Design review of the part built by this model. Coordinates are the model's own, in mm. A direction names the side the tool comes from. Round coordinates to 2 decimals unless told otherwise and drop trailing zeros. Order: outer loops, then holes, each group sorted by start corner. A loop starts at its lowest first (then second) coordinate and runs counter-clockwise, first axis right, second up. Notation, with made-up numbers: (-8, -30) - (-4, -30) arc R21 ccw to (-4, 2) - close; hole circle Ø9 at (-24, 14.25). An arc over 180 degrees is marked (long way). Write item = value, one per line.
from build123d import *
from build123d import SkipClean  # not in build123d's __all__

# Parameters (mm, degrees)
F0_R     = 26
F1_DEPTH = 8
F2_R     = 26.25
F2_R_2   = 20
F3_DEPTH = 82.5


with BuildPart() as f1:
    # F0 (on Top) → F1 (new body)
    with BuildSketch(Plane.XY):
        Circle(F0_R)
        with BuildLine():
            ThreePointArc((7, 18.7349939952), (19.9390246123, -1.5605439791), (4, -19.5959179423))
            Line((4, -19.5959179423), (2.5, -16.9978417309))
            ThreePointArc((2.5, -16.9978417309), (0, -17.1816769299), (-2.5, -16.9978417309))
            Line((-2.5, -16.9978417309), (-4, -19.5959179423))
            ThreePointArc((-4, -19.5959179423), (-19.9390246123, -1.5605439791), (-7, 18.7349939952))
            Line((-7, 18.7349939952), (-5, 16.4989260177))
            ThreePointArc((-5, 16.4989260177), (0, 17.2452185999), (5, 16.4989260177))
            Line((5, 16.4989260177), (7, 18.7349939952))
        make_face(mode=Mode.SUBTRACT)
    extrude(amount=F1_DEPTH)

    # F2 (on face) → F3 (join)
    with BuildSketch(Plane.XY.offset(8)):
        Circle(F2_R)
        Circle(F2_R_2, mode=Mode.SUBTRACT)
    with SkipClean():  # cleaning this boolean's faces spoils the solid; the shape is the same uncleaned
        extrude(amount=F3_DEPTH)


solid = f1.part
1) Clearance check with flat-ended pins moving along their axes: pin 1 Ø3 at (x, z) = (6, 47.5) entering from -Y; pin 2 Ø4 at (y, z) = (-11, 64.5) entering from +X; pin 3 Ø3 at (y, z) = (3, 35.5) entering from -X. State where each tip first meets the part, or that it passes through.
Findings:
pin_1 = -25.86
pin_2 = 24.66
pin_3 = -26.21
2) For faces 5 (the cylindrical face through (-20.633, -15.821, 3.944)), 6 (the flat face through (-6, -19.3, 90.5)), 7 (the cylindrical face through (0.04, -17.18, 3.94)), 8 (the flat face through (0, -18, 8)), list the 3-axis set-ups (+Z, -Z, +X, -X, +Y, -Y) from which the entire face can be reached by the end or side of a thin tool; tool diameter is ignored.
Findings:
face_5 = -Z
face_6 = +Z, +X, -X, +Y, -Y
face_7 = +Z, -Z
face_8 = +Z
3) We need section A-A on y = 0. Write out the cut boundary in (x, z), and give its area (3 significant figures).
Findings:
outline = (-26.25, 8) - (-26, 8) - (-26, 0) - (-20, 0) - (-20, 90.5) - (-26.25, 90.5) - close; (20, 0) - (26, 0) - (26, 8) - (26.25, 8) - (26.25, 90.5) - (20, 90.5) - close
area = 1,130 mm^2
4) We need section C-C on z = 63. Write out the cut boundary in (x, y).
Findings:
outline = circle Ø52.5 at (0, 0); hole circle Ø40 at (0, 0)
5) To check wall thickness, follow L1, parallel to Y at x = 0, z = 31.5; L2, parallel to X at y = 17.5, z = 5; L3, parallel to X at y = 0.5, z = 61. State the ranges of each line that lie inside material, in increasing order. Write a range as from..to.
Findings:
L1 = -26.25..-20, 20..26.25
L2 = -19.23..-9.68, -5.9..5.9, 9.68..19.23
L3 = -26.25..-19.99, 19.99..26.25
6) We need section B-B on x = 0. Write out the cut boundary in (y, z).
Findings:
outline = (-26.25, 8) - (-26, 8) - (-26, 0) - (-17.18, 0) - (-17.18, 8) - (-20, 8) - (-20, 90.5) - (-26.25, 90.5) - close; (17.25, 0) - (26, 0) - (26, 8) - (26.25, 8) - (26.25, 90.5) - (20, 90.5) - (20, 8) - (17.25, 8) - close
7) The part is to be moulded in two halves that separate along Y. For faces 1 (the flat face through (-3.24, -18.28, 3.94)), 2 (the cylindrical face through (25, 8, 49)), 3 (the flat face through (0, 18, 8)), 4 (the flat face through (0, 18, 0)), say which applies: released by +Y, released by -Y, zero draft, split by the parting line, or undercut.
Findings:
face_1 = undercut
face_2 = split by the parting line
face_3 = undercut
face_4 = zero draft
8) We need section D-D on x = -21.5. Write out the cut boundary in (y, z).
Findings:
outline = (-15.06, 8) - (-14.62, 8) - (-14.62, 0) - (14.62, 0) - (14.62, 8) - (15.06, 8) - (15.06, 90.5) - (-15.06, 90.5) - close
